from build123d import *

# Parameters (mm, degrees)
F0_R     = 11.4
F1_DEPTH = 7.5
F2_R     = 1.5
F3_SIZE  = 1


with BuildPart() as f1:
    # F0 (on Top) → F1 (new body)
    with BuildSketch(Plane.XY):
        with BuildLine():
            Line((15.4, 12.557368), (15.4, 29))
            ThreePointArc((15.4, 29), (0, 44.4), (-15.4, 29))
            Line((-15.4, 29), (-15.4, 12.557368))
            ThreePointArc((-15.4, 12.557368), (-16.250739, 9.382368), (-18.575, 7.058107))
            Line((-18.575, 7.058107), (-32.814737, -1.163209))
            ThreePointArc((-32.814737, -1.163209), (-38.451528, -22.2), (-17.414737, -27.836791))
            Line((-17.414737, -27.836791), (-3.175, -19.615475))
            ThreePointArc((-3.175, -19.615475), (0, -18.764737), (3.175, -19.615475))
            Line((3.175, -19.615475), (17.414737, -27.836791))
            ThreePointArc((17.414737, -27.836791), (38.451528, -22.2), (32.814737, -1.163209))
            Line((32.814737, -1.163209), (18.575, 7.058107))
            ThreePointArc((18.575, 7.058107), (16.250739, 9.382368), (15.4, 12.557368))
        make_face()
        with Locations((-25.114737, -14.5)):
            Circle(F0_R, mode=Mode.SUBTRACT)
        with Locations((25.114737, -14.5)):
            Circle(F0_R, mode=Mode.SUBTRACT)
        Circle(F0_R, mode=Mode.SUBTRACT)
        with Locations((0, 29)):
            Circle(F0_R, mode=Mode.SUBTRACT)
    extrude(amount=F1_DEPTH)

    # F2
    f2_edges = [f1.edges().sort_by_distance(p)[0] for p in [
        (-16.250739, 9.382368, 0),
        (15.4, 12.557368, 3.75),
        (25.694868, 2.947449, 7.5),
    ]]
    fillet(f2_edges, radius=F2_R)

    # F3
    f3_edges = [f1.edges().sort_by_distance(p)[0] for p in [
        (-11.4, 29, 7.5),
        (-11.4, 0, 0),
        (-11.4, 0, 7.5),
        (13.714737, -14.5, 0),
        (13.714737, -14.5, 7.5),
        (-36.514737, -14.5, 7.5),
        (-36.514737, -14.5, 0),
        (-11.4, 29, 0),
    ]]
    chamfer(f3_edges, length=F3_SIZE)


solid = f1.part
Design review of the part built by this model. Coordinates are the model's own, in mm. A direction names the side the tool comes from. Round coordinates to 2 decimals unless told otherwise and drop trailing zeros. Write each loop counter-clockwise with the first axis right and the second up, starting at its lowest first coordinate (ties: lowest second). Pieces come first, ordered by that corner, then holes. Notation, with made-up numbers: (72, 30.5) -> (113, 30.5) arc R10 cw to (113, 36.5) -> close; hole circle Ø4 at (-2.75, 4.25). An arc over 180 degrees is marked (long way). One line per item, written item: value. Start each with the question number.
Q1. Insertion check: P1, Ø1.3, axis at y = 17.5, z = 3, coming from the -X side; P2, Ø2, axis at y = -7.5, z = 6, coming from the -X side; P3, Ø1, axis at x = 9, z = 3.5, coming from the -Y side. Each pin has a flat end and moves straight along its axis. Give the tip position at first contact, or say it passes through.
Q2. Add section B-B (x = 0). Give the boundary of the cut face in (y, z).
Q3. Add section C-C (z = 5). Give the boundary of the cut face in (x, y) (3 decimals), then the cut area to 3 significant figures.
Q4. Add section A-A (y = -14.5). Give the boundary of the cut face in (x, z).
Q5. To check wall thickness, follow probe 1 along X at (y, z) = (-15, 5.25); probe 2 along Y at (x, z) = (0, 3.05); probe 3 along Y at (x, z) = (-10, 4.25). State the ranges of each line that lie inside material, in increasing order.
Q6. Tool access review of faces 4 (the face through (10.61, -23.41, 0.45)), 5 (the face through (-10.39, -23.78, 3.72)), 6 (the face through (-15.4, 21, 4)): name each direction out of +Z, -Z, +X, -X, +Y, -Y from which nothing blocks a thin tool from reaching the whole face with its end or side.
Q7. The part is to be moulded in two halves that separate along Y. For faces 1 (the face through (0.339, 44.396, 3.718)), 2 (the face through (13.726, -13.999, 3.712)), 3 (the face through (10.61, -23.41, 7.05)), say which applies: pulls with the +Y half, pulls with the -Y half, needs draft (parallel to the pull), parting line crosses it, or undercut.
Response:
1. P1: stops at x = -15.4
1. P2: stops at x = -39.3
1. P3: stops at y = -23.27
2. outline: (-18.76, 1.5) arc R1.5 ccw to (-17.26, 0) -> (-12.4, 0) -> (-11.4, 1) -> (-11.4, 6.5) -> (-12.4, 7.5) -> (-17.26, 7.5) arc R1.5 ccw to (-18.76, 6) -> close; (11.4, 1) -> (12.4, 0) -> (16.6, 0) -> (17.6, 1) -> (17.6, 6.5) -> (16.6, 7.5) -> (12.4, 7.5) -> (11.4, 6.5) -> close; (40.4, 1) -> (41.4, 0) -> (42.9, 0) arc R1.5 ccw to (44.4, 1.5) -> (44.4, 6) arc R1.5 ccw to (42.9, 7.5) -> (41.4, 7.5) -> (40.4, 6.5) -> close
3. outline: (-32.815, -1.163) arc R15.4 ccw to (-17.415, -27.837) -> (-3.175, -19.615) arc R6.35 cw to (3.175, -19.615) -> (17.415, -27.837) arc R15.4 ccw to (32.815, -1.163) -> (18.575, 7.058) arc R6.35 cw to (15.4, 12.557) -> (15.4, 29) arc R15.4 ccw to (-15.4, 29) -> (-15.4, 12.557) arc R6.35 cw to (-18.575, 7.058) -> close; hole circle Ø22.8 at (-25.115, -14.5); hole circle Ø22.8 at (0, 0); hole circle Ø22.8 at (0, 29); hole circle Ø22.8 at (25.115, -14.5)
3. area: 1,760 mm^2
4. outline: (-40.51, 1.5) arc R1.5 ccw to (-39.01, 0) -> (-37.51, 0) -> (-36.51, 1) -> (-36.51, 6.5) -> (-37.51, 7.5) -> (-39.01, 7.5) arc R1.5 ccw to (-40.51, 6) -> close; (-13.71, 1) -> (-12.71, 0) -> (12.71, 0) -> (13.71, 1) -> (13.71, 6.5) -> (12.71, 7.5) -> (-12.71, 7.5) -> (-13.71, 6.5) -> close; (36.51, 1) -> (37.51, 0) -> (39.01, 0) arc R1.5 ccw to (40.51, 1.5) -> (40.51, 6) arc R1.5 ccw to (39.01, 7.5) -> (37.51, 7.5) -> (36.51, 6.5) -> close
5. probe 1: x = -40.51 to -36.5, -13.73 to 13.73, 36.5 to 40.51
5. probe 2: y = -18.76 to -11.4, 11.4 to 17.6, 40.4 to 44.4
5. probe 3: y = -23.56 to -5.47, 5.47 to 23.53, 34.47 to 40.71
6. face 4: -Z, -Y
6. face 5: +Z, -Z, -Y
6. face 6: +Z, -Z, -X, +Y
7. face 1: pulls with the +Y half
7. face 2: undercut
7. face 3: pulls with the -Y half
